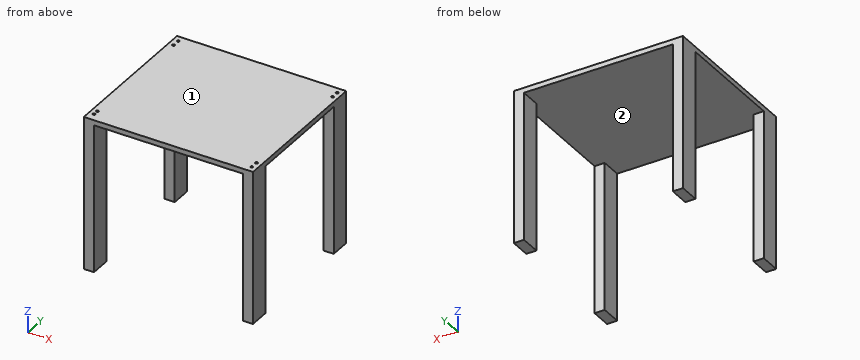
```python
from build123d import *

# Parameters (mm, degrees)
F0_W     = 400
F0_H     = 360
F0_R     = 3
F2_DEPTH = 12
F1_W     = 24
F1_H     = 48
F3_DEPTH = 350


with BuildPart() as f2:
    # F0 (on Top) → F2 (new body)
    with BuildSketch(Plane.XY):
        with Locations((-30.968213, -48.251697)):
            Rectangle(F0_W, F0_H)
        with Locations((-218.968213, -208.251697)):
            Circle(F0_R, mode=Mode.SUBTRACT)
        with Locations((-218.968213, -195.251697)):
            Circle(F0_R, mode=Mode.SUBTRACT)
        with Locations((157.031787, -213.251697)):
            Circle(F0_R, mode=Mode.SUBTRACT)
        with Locations((157.031787, -195.251697)):
            Circle(F0_R, mode=Mode.SUBTRACT)
        with Locations((-218.968213, 98.748303)):
            Circle(F0_R, mode=Mode.SUBTRACT)
        with Locations((-218.968213, 116.748303)):
            Circle(F0_R, mode=Mode.SUBTRACT)
        with Locations((157.031787, 98.748303)):
            Circle(F0_R, mode=Mode.SUBTRACT)
        with Locations((157.031787, 116.748303)):
            Circle(F0_R, mode=Mode.SUBTRACT)
    extrude(amount=F2_DEPTH)

    # F1 (on Top) → F3 (join)
    with BuildSketch(Plane.XY):
        with Locations((-218.968213, -204.251697)):
            Rectangle(F1_W, F1_H)
        with Locations((-218.968213, 107.748303)):
            Rectangle(F1_W, F1_H)
        with Locations((157.031787, 107.748303)):
            Rectangle(F1_W, F1_H)
        with Locations((157.031787, -204.251697)):
            Rectangle(F1_W, F1_H)
    extrude(amount=-F3_DEPTH)


solid = f2.part
```
Geometry check sheet. Reference: the model listing, model coordinates, mm. Face numbers are marked on the shaded views. Coordinates: 2 decimals unless noted, no trailing zeros. Order: outer loops, then holes, each group sorted by start corner. A loop starts at its lowest first (then second) coordinate and runs counter-clockwise, first axis right, second up.
Q1. Sectioned sample at C-C on y = -2. Record the cut outline in (x, z), and give its area (3 significant figures).
Reply:
outline: (-230.97, 0) - (169.03, 0) - (169.03, 12) - (-230.97, 12) - close
area: 4,800 mm2
Q2. Sectioned sample at B-B on x = 127. Record the cut outline in (y, z), and give its area (3 significant figures).
Reply:
outline: (-228.25, 0) - (131.75, 0) - (131.75, 12) - (-228.25, 12) - close
area: 4,320 mm2
Q3. Thickness scan on probe 1 along X at (y, z) = (-208, -322); probe 2 along Y at (x, z) = (151, -289); probe 3 along Z at (x, y) = (-126.5, -49.5). Record the ranges inside material, lowest first.
Reply:
probe 1: x = -230.97 to -206.97, 145.03 to 169.03
probe 2: y = -228.25 to -180.25, 83.75 to 131.75
probe 3: z = 0 to 12
Q4. Depth check by flat-ended pin: pin 1 Ø3 at (x, y) = (157.5, -214.5) entering from +Z; pin 2 Ø1 at (x, y) = (-53, -163) entering from -Z; pin 3 Ø12 at (y, z) = (-168.5, -218) entering from +X (1 decimal). Enter the tip coordinate at first touch or a pass-through.
Reply:
pin 1: stops at z = 0
pin 2: stops at z = 0
pin 3: passes through
Q5. Draft check along X on the marked faces 1 and 2. Enter one of: released by +X, released by -X, zero draft, split by the parting line, or undercut.
Reply:
face 1: zero draft
face 2: undercut
Q6. Sectioned sample at A-A on z = -279. Record the cut outline in (x, y).
Reply:
outline: (-230.97, -228.25) - (-206.97, -228.25) - (-206.97, -180.25) - (-230.97, -180.25) - close; (-230.97, 83.75) - (-206.97, 83.75) - (-206.97, 131.75) - (-230.97, 131.75) - close; (145.03, -228.25) - (169.03, -228.25) - (169.03, -180.25) - (145.03, -180.25) - close; (145.03, 83.75) - (169.03, 83.75) - (169.03, 131.75) - (145.03, 131.75) - close
